from build123d import *

# Parameters (mm, degrees)
SKETCH1_R      = 4.191
EXTRUDE1_DEPTH = 0.7874
EXTRUDE2_DEPTH = 3.85318
SKETCH3_R      = 2.38125
EXTRUDE3_DEPTH = 8.069367589


with BuildPart() as part:
    # Sketch1 → Extrude1 (new body)
    with BuildSketch(Plane.XY):
        Circle(SKETCH1_R)
    extrude(amount=EXTRUDE1_DEPTH)

    # Sketch2 → Extrude2 (add)
    with BuildSketch(Plane.XY):
        Polygon((-0.265291692, -3.656563093), (3.034030683, -2.058030891), (3.299322375, 1.598532202), (0.265291692, 3.656563093), (-3.034030683, 2.058030891), (-3.299322375, -1.598532202), align=None)
    extrude(amount=EXTRUDE2_DEPTH)

    # Sketch3 → Extrude3 (cut, through all)
    with BuildSketch(Plane(origin=(0, 0, 0), x_dir=(-1, 0, 0), z_dir=(0, 0, -1))):
        Circle(SKETCH3_R)
    extrude(amount=-EXTRUDE3_DEPTH, mode=Mode.SUBTRACT)


solid = part.part
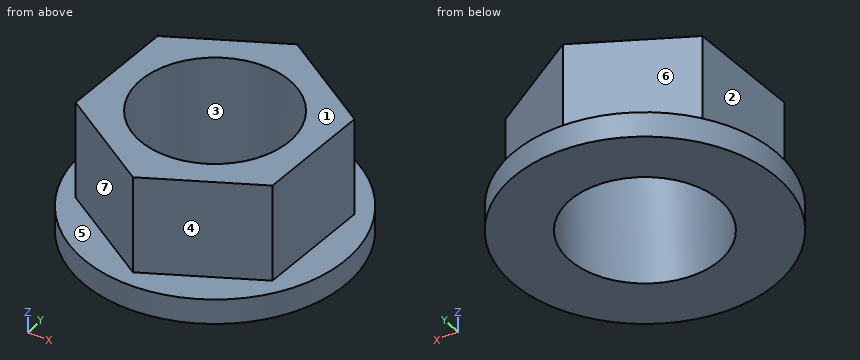
Check sheet for the modelled part. Datum: model origin and axes. Units: mm. Face numbers are marked on the shaded views. A direction names the side the tool comes from. Give positions to 0.01 mm unless a question says otherwise; leave off trailing zeros. Loops run counter-clockwise (first coordinate to the right, second up) from the corner with the lowest first, then second, coordinate; pieces in that order, holes last. Notation, with made-up numbers: M 84,38 L 136,38 A28 ccw 136,70 Z; hole C -15.75,10.25 d11. An arc over 180 degrees is marked long. Answer as a JSON object with one key per item and string values. Group by question number.
Q1. Access from +Z, -Z, +X, -X, +Y, -Y to the whole of each face (thin tool, end or side, straight path). Record for the marked faces 4, 5, 6 and 7.
Q2. Cross-section at D-D on x = -2.75. Record the cut outline in (y, z), then the cut area to 3 significant figures.
Q3. Cross-section at B-B on z = 2.85. Record the cut outline in (x, y).
Q4. Cross-section at A-A on x = 0.75. Record the cut outline in (y, z).
Q5. Cross-section at C-C on y = 0. Record the cut outline in (x, z), then the cut area to 3 significant figures.
Q6. Release check for a two-part mould opening along Y. For the marked faces 1, 2 and 3 record: released by +Y, released by -Y, zero draft, split by the parting line, or undercut.
Q7. Material ranges on line 1 along Y through (x, z) = (0, 0.65); line 2 along X through (y, z) = (-1.5, 3.3); line 3 along Y through (x, z) = (0, 1.6), recorded low to high. Write a range as [from, to].
Q8. Go/stop test with flat-tipped pins: P1, Ø1, axis at x = -2, z = 2, coming from the -Y side; P2, Ø1.5, axis at x = -3, y = -3, coming from the +Z side; P3, Ø1.5, axis at y = 0, z = 2.5, coming from the +X side; P4, Ø4, axis at x = 0, y = 0, coming from the -Z side. Record where each tip stops, or that it passes through.
Evaluation:
{
 "1": {"face 4": "+Z, +X, -Y", "face 5": "+Z", "face 6": "+Z, -X, +Y", "face 7": "+Z, -X, -Y"},
 "2": {"outline": "M -3.16,0 L 3.16,0 L 3.16,0.79 L 2.2,0.79 L 2.2,3.85 L -1.97,3.85 L -1.97,0.79 L -3.16,0.79 Z", "area": "17.8 mm2"},
 "3": {"outline": "M -3.3,-1.6 L -0.27,-3.66 L 3.03,-2.06 L 3.3,1.6 L 0.27,3.66 L -3.03,2.06 Z; hole C 0,0 d4.76"},
 "4": {"outline": "M -4.12,0 L -2.26,0 L -2.26,3.85 L -3.16,3.85 L -3.16,0.79 L -4.12,0.79 Z; M 2.26,0 L 4.12,0 L 4.12,0.79 L 3.33,0.79 L 3.33,3.85 L 2.26,3.85 Z"},
 "5": {"outline": "M -4.19,0 L -2.38,0 L -2.38,3.85 L -3.18,3.85 L -3.18,0.79 L -4.19,0.79 Z; M 2.38,0 L 4.19,0 L 4.19,0.79 L 3.18,0.79 L 3.18,3.85 L 2.38,3.85 Z", "area": "7.77 mm2"},
 "6": {"face 1": "zero draft", "face 2": "released by +Y", "face 3": "undercut"},
 "7": {"line 1": "y = [-4.19, -2.38], [2.38, 4.19]", "line 2": "x = [-3.29, -1.85], [1.85, 3.07]", "line 3": "y = [-3.53, -2.38], [2.38, 3.53]"},
 "8": {"P1": "stops at y = -2.82", "P2": "stops at z = 0.79", "P3": "stops at x = 3.24", "P4": "passes through"}
}
